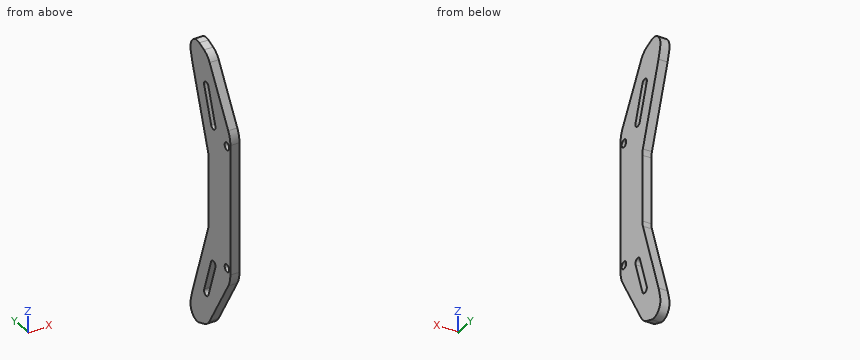
```python
from build123d import *

# Parameters (mm, degrees)
BOSS_EXTRUDE1_DEPTH = 6.35
SLOTS_DEPTH         = 7.3500001
SKETCH3_R           = 2.65
HOLES_DEPTH         = 7.3500001
FILLET1_R           = 12.7
FILLET2_R           = 17.78


with BuildPart() as part:
    # Sketch1 → Boss-Extrude1 (new body)
    with BuildSketch(Plane(origin=(0, 0, 0), x_dir=(0, 0, -1), z_dir=(1, 0, 0))):
        with BuildLine():
            Line((50.8, 0), (-50.8, 0))
            Line((-50.8, 0), (-95.491911785, 26.510580519))
            Line((-95.491911785, 26.510580519), (-99.095159206, 36.267222623))
            add(Edge.make_bspline(
                [(-81.095679658, 44.383857392), (-84.793404741, 45.36773864), (-94.554651266, 49.479684382), (-100.787803101, 40.484157915), (-99.095159206, 36.267222623)],
                knots=[0, 0, 0, 0, 0.528781937, 1, 1, 1, 1], degree=3))
            Line((-81.095679658, 44.383857392), (-25.4, 25.4))
            Line((-25.4, 25.4), (25.4, 25.4))
            Line((25.4, 25.4), (81.095679658, 44.383857392))
            add(Edge.make_bspline(
                [(81.095679658, 44.383857392), (84.793404741, 45.36773864), (94.554651266, 49.479684382), (100.787803101, 40.484157915), (99.095159206, 36.267222623)],
                knots=[0, 0, 0, 0, 0.528781937, 1, 1, 1, 1], degree=3))
            Line((99.095159206, 36.267222623), (95.491911785, 26.510580519))
            Line((95.491911785, 26.510580519), (50.8, 0))
        make_face()
    extrude(amount=BOSS_EXTRUDE1_DEPTH)

    # Sketch2 → slots (cut, through all)
    with BuildSketch(Plane.ZY):
        with BuildLine():
            Line((-72.404954671, 30.615105796), (-48.363160058, 22.420466586))
            ThreePointArc((-48.363160058, 22.420466586), (-46.741010292, 19.120674147), (-50.040802731, 17.498524382))
            Line((-50.040802731, 17.498524382), (-74.082597344, 25.693163592))
            ThreePointArc((-74.082597344, 25.693163592), (-75.70474711, 28.992956031), (-72.404954671, 30.615105796))
        make_face()
        with BuildLine():
            Line((72.404954671, 30.615105796), (48.363160058, 22.420466586))
            ThreePointArc((48.363160058, 22.420466586), (46.741010292, 19.120674147), (50.040802731, 17.498524382))
            Line((50.040802731, 17.498524382), (74.082597344, 25.693163592))
            ThreePointArc((74.082597344, 25.693163592), (75.70474711, 28.992956031), (72.404954671, 30.615105796))
        make_face()
    extrude(amount=-SLOTS_DEPTH, mode=Mode.SUBTRACT)

    # Sketch3 → holes (cut, through all)
    with BuildSketch(Plane.ZY):
        with Locations((-43.18, 4)):
            Circle(SKETCH3_R)
        with Locations((43.18, 4)):
            Circle(SKETCH3_R)
    extrude(amount=-HOLES_DEPTH, mode=Mode.SUBTRACT)

    # Fillet1
    fillet1_edges = [part.edges().sort_by_distance(p)[0] for p in [
        (3.175, 26.510580519, 95.491911785),
        (3.175, 25.4, 25.4),
        (3.175, 25.4, -25.4),
        (3.175, 26.510580519, -95.491911785),
    ]]
    fillet(fillet1_edges, radius=FILLET1_R)

    # Fillet2
    fillet2_edges = [part.edges().sort_by_distance(p)[0] for p in [
        (3.175, 0, -50.8),
        (3.175, 0, 50.8),
    ]]
    fillet(fillet2_edges, radius=FILLET2_R)


solid = part.part
```
Can you work these out from the model? Positions are in its coordinate system, mm. Coordinates: 2 decimals unless noted, no trailing zeros. Order: outer loops, then holes, each group sorted by start corner. A loop starts at its lowest first (then second) coordinate and runs counter-clockwise, first axis right, second up. Notation, with made-up numbers: (-30.5, 13) -> (19.5, 13) arc R5 ccw to (19.5, 19) -> close; hole circle Ø5 at (89, 13). An arc over 180 degrees is marked (long way). Write each question's results on one line, items separated by ' | '.
Item 1: If I drill on line 1 along Z through (x, y) = (4, 3.5); line 2 along Y through (x, z) = (4.5, 50.5); line 3 along Y through (x, z) = (3, 59), over which ranges is the centre line in solid material (lowest first)?
Results are:
line 1: -56.7 to -45.78, -40.58 to 40.58, 45.78 to 56.7 | line 2: 0.6 to 17.66, 23.15 to 33.96 | line 3: 4.86 to 20.55, 26.05 to 36.85
Item 2: I'm going to push flat-ended pins straight in: pin 1 Ø2 at (x, y) = (0.5, 13.5) entering from +Z; pin 2 Ø2 at (x, z) = (2, -75) entering from -Y. Where does each tip first touch, or does it pass through?
Results are:
pin 1: z = 75.24 | pin 2: y = 13.76
Item 3: I want a section at D-D, the plane x = 3.25. Count the separate pieces of the cut face and the enclosed holes in it, then the cut area to 3 significant figures.
Results are:
separate pieces: 1 | enclosed holes: 4 | area: 5,050 mm²
Item 4: I want a section at A-A, the plane y = 19.5. Write out the boundary of the cut face in (x, z), then the cut area to 3 significant figures.
Results are:
outline: (0, -83.67) -> (6.35, -83.67) -> (6.35, -55.91) -> (0, -55.91) -> close; (0, -46.64) -> (6.35, -46.64) -> (6.35, 46.64) -> (0, 46.64) -> close; (0, 55.91) -> (6.35, 55.91) -> (6.35, 83.67) -> (0, 83.67) -> close | area: 945 mm²
Item 5: I want a section at C-C, the plane y = 32.5. Write out the boundary of the cut face in (x, z).
Results are:
outline: (0, -97.7) -> (6.35, -97.7) -> (6.35, -46.23) -> (0, -46.23) -> close; (0, 46.23) -> (6.35, 46.23) -> (6.35, 97.7) -> (0, 97.7) -> close
Item 6: I want a section at B-B, the plane z = 65.5. Write out the boundary of the cut face in (x, y), then the cut area to 3 significant figures.
Results are:
outline: (0, 8.72) -> (6.35, 8.72) -> (6.35, 22.77) -> (0, 22.77) -> close; (0, 28.26) -> (6.35, 28.26) -> (6.35, 39.07) -> (0, 39.07) -> close | area: 158 mm²
